```python
from build123d import *

# Parameters (mm, degrees)
BOSS_EXTRUDE1_DEPTH = 10
SKETCH2_R           = 1.75
CUT_EXTRUDE1_DEPTH  = 14
CHAMFER1_SIZE       = 1.5
CHAMFER3_SIZE       = 0.5


with BuildPart() as part:
    # Sketch1 → Boss-Extrude1 (new body, symmetric)
    with BuildSketch(Plane.XY):
        Polygon((0, 0), (15, 0), (15, 6), (10, 6), (10, 9), (15, 9), (15, 13), (0, 13), (0, 9), (5, 9), (5, 6), (0, 6), align=None)
    extrude(amount=BOSS_EXTRUDE1_DEPTH, both=True)

    # Sketch2 → Cut-Extrude1 (cut, through all)
    with BuildSketch(Plane(origin=(0, 13, 0), x_dir=(1, 0, 0), z_dir=(0, 1, 0))):
        with Locations((7.5, -5)):
            Circle(SKETCH2_R)
        with Locations((7.5, 5)):
            Circle(SKETCH2_R)
    extrude(amount=-CUT_EXTRUDE1_DEPTH, mode=Mode.SUBTRACT)

    # Chamfer1
    chamfer1_edges = [part.edges().sort_by_distance(p)[0] for p in [
        (0, 13, 0),
        (15, 13, 0),
    ]]
    chamfer(chamfer1_edges, length=CHAMFER1_SIZE)

    # Chamfer3
    chamfer3_edges = [part.edges().sort_by_distance(p)[0] for p in [
        (5.75, 13, 5),
        (5.75, 13, -5),
    ]]
    chamfer(chamfer3_edges, length=CHAMFER3_SIZE)


solid = part.part
```
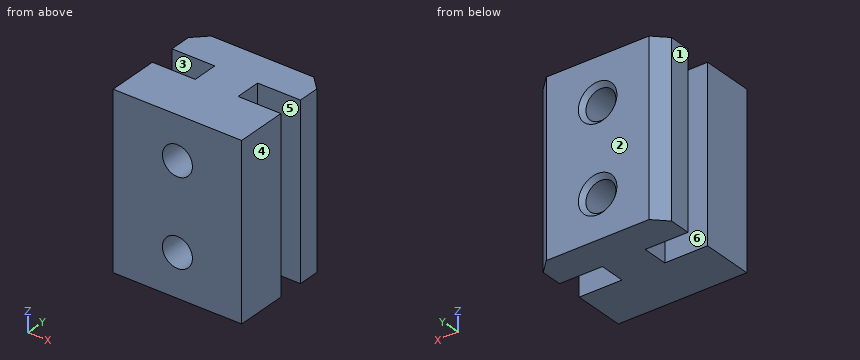
CAD build for the part. Positions are in the model's coordinates, mm. Face numbers are marked on the shaded views. A direction names the side the tool comes from. Coordinates: 2 decimals unless noted, no trailing zeros. Write each loop counter-clockwise with the first axis right and the second up, starting at its lowest first coordinate (ties: lowest second). Pieces come first, ordered by that corner, then holes. Notation, with made-up numbers: (4.25, 23.5) -> (36.25, 23.5) arc R33 ccw to (36.25, 61.5) -> close; hole circle Ø11 at (39, 46). An arc over 180 degrees is marked (long way). Return JSON: item names as keys, results as strings. Group by question number.
Q1. Which spindle directions (+Z, -Z, +X, -X, +Y, -Y) get a long thin tool onto all of the face, cutting with end or side? Do the marked faces 4, 5 and 6. Say none if no direction does.
Q2. Flat gauge pins, fed straight in: pin 1 (3 mm diameter, centred on x = 7.5, z = -5, fed in from -Y) (3 decimals); pin 2 (1.5 mm diameter, centred on y = 7.5, z = 2, fed in from +X). Where does each tip first touch, or does it go through?
Q3. Cut at D-D, the plane z = 1. Give the cut face in (x, y).
Q4. Cut at C-C, the plane y = 8.75. Give the cut face in (x, z), then the cut area to 3 significant figures.
Q5. Cut at A-A, the plane x = 7.5. Give the cut face in (y, z).
Q6. Cut at B-B, the plane z = -5. Give the cut face in (x, y).
Q7. Pull direction Y, two halves, no side cores. Call the marked faces 1, 2 and 3: released by +Y, released by -Y, zero draft, split by the parting line, or undercut.
Q8. Drill centre lines: line 1 (Z direction, x = 7.5, y = 7); line 2 (Y direction, x = 3.75, z = 5); line 3 (Z direction, x = 8.75, y = 8). Where is each one in solid material? Low to high.
Returned:
{
 "1": {"face 4": "+Z, -Z, +X, +Y, -Y", "face 5": "+Z, -Z, +X", "face 6": "+Z, -Z, -X"},
 "2": {"pin 1": "passes through", "pin 2": "stops at x = 10"},
 "3": {"outline": "(0, 0) -> (15, 0) -> (15, 6) -> (10, 6) -> (10, 9) -> (15, 9) -> (15, 11.5) -> (13.5, 13) -> (1.5, 13) -> (0, 11.5) -> (0, 9) -> (5, 9) -> (5, 6) -> (0, 6) -> close"},
 "4": {"outline": "(5, -10) -> (10, -10) -> (10, 10) -> (5, 10) -> close; hole circle Ø3.5 at (7.5, -5); hole circle Ø3.5 at (7.5, 5)", "area": "80.8 mm2"},
 "5": {"outline": "(0, -10) -> (13, -10) -> (13, -7.25) -> (12.5, -6.75) -> (0, -6.75) -> close; (0, -3.25) -> (12.5, -3.25) -> (13, -2.75) -> (13, 2.75) -> (12.5, 3.25) -> (0, 3.25) -> close; (0, 6.75) -> (12.5, 6.75) -> (13, 7.25) -> (13, 10) -> (0, 10) -> close"},
 "6": {"outline": "(0, 0) -> (5.75, 0) -> (5.75, 12.5) -> (5.25, 13) -> (1.5, 13) -> (0, 11.5) -> (0, 9) -> (5, 9) -> (5, 6) -> (0, 6) -> close; (9.25, 0) -> (15, 0) -> (15, 6) -> (10, 6) -> (10, 9) -> (15, 9) -> (15, 11.5) -> (13.5, 13) -> (9.75, 13) -> (9.25, 12.5) -> close"},
 "7": {"face 1": "zero draft", "face 2": "released by +Y", "face 3": "undercut"},
 "8": {"line 1": "z = -10 to -6.75, -3.25 to 3.25, 6.75 to 10", "line 2": "y = 0 to 6, 9 to 13", "line 3": "z = -10 to -6.22, -3.78 to 3.78, 6.22 to 10"}
}
